Source: CAD feature listing. Evaluate the final solid. Frame: model axes, mm. Coordinates: 2 decimals unless noted, no trailing zeros. Order: outer loops, then holes, each group sorted by start corner. A loop starts at its lowest first (then second) coordinate and runs counter-clockwise, first axis right, second up. Notation, with made-up numbers: (80.5, -35.5) -> (124.5, -35.5) arc R19 ccw to (124.5, -11.5) -> close; hole circle Ø2 at (41, -20.5). An arc over 180 degrees is marked (long way). Put each result on its own line as item: value.
Autodesk Inventor part; units mm, degrees
ref_plane "YZ Plane" through (0, 0, 0) normal (1, 0, 0) x (0, 1, 0)
ref_plane "XZ Plane" through (0, 0, 0) normal (0, 1, 0) x (-1, 0, 0)
ref_plane "XY Plane" through (0, 0, 0) normal (0, 0, 1) x (1, 0, 0)
sketch "Sketch1" plane through (0, 0, 0) normal (0, 0, 1) x (1, 0, 0)
  line L0 (-8.0811, -5.1131) -> (16.9189, -5.1131)
  line L1 (16.9189, -5.1131) -> (16.9189, 19.8869)
  line L2 (16.9189, 19.8869) -> (-8.0811, 19.8869)
  line L3 (-8.0811, 19.8869) -> (-8.0811, -5.1131)
  line L4 (-8.0811, -5.1131) -> (-7.0811, -5.1131)
  line L5 (-7.0811, -5.1131) -> (-7.0811, -4.1131)
  line L6 (-7.0811, -4.1131) -> (-8.0811, -4.1131)
  line L7 (-8.0811, -4.1131) -> (-8.0811, -5.1131)
  line L8 (16.9189, 19.8869) -> (15.9189, 19.8869)
  line L9 (15.9189, 19.8869) -> (15.9189, 18.8869)
  line L10 (15.9189, 18.8869) -> (16.9189, 18.8869)
  line L11 (16.9189, 18.8869) -> (16.9189, 19.8869)
  line L12 (-7.0811, -4.1131) -> (15.9189, -4.1131)
  line L13 (15.9189, -4.1131) -> (15.9189, 18.8869)
  line L14 (15.9189, 18.8869) -> (-7.0811, 18.8869)
  line L15 (-7.0811, 18.8869) -> (-7.0811, -4.1131)
  line L16 (-7.0811, -4.1131) -> (-1.0811, -4.1131)
  line L17 (-1.0811, -4.1131) -> (-1.0811, 17.1845)
  line L18 (-1.0811, 17.1845) -> (-7.0811, 17.1845)
  line L19 (-7.0811, 17.1845) -> (-7.0811, -4.1131)
  line L20 (15.9189, -4.1131) -> (9.9189, -4.1131)
  line L21 (9.9189, -4.1131) -> (9.9189, 17.1845)
  line L22 (9.9189, 17.1845) -> (15.9189, 17.1845)
  line L23 (15.9189, 17.1845) -> (15.9189, -4.1131)
  circle A0 centre (4.4189, 0.3869) radius 5.5
  line L24 (4.4189, 0.3869) -> (15.9189, 0.3869)
  line L25 (4.4189, 0.3869) -> (-8.0811, 0.3869)
  circle A1 centre (-4.0811, 3.3869) radius 3
  circle A2 centre (12.9189, 3.3869) radius 3
  circle A3 centre (4.4189, 0.3869) radius 5
  line L26 (4.4189, -4.6131) -> (4.4189, -3.3131)
  line L27 (4.4189, -3.3131) -> (16.9189, -3.3131)
  line L28 (4.4189, -3.3131) -> (-8.0811, -3.3131)
  line L29 (-4.0811, 6.3869) -> (-4.0811, 8.3869)
  line L30 (-4.0811, 8.3869) -> (16.9189, 8.3869)
  line L31 (-4.0811, 8.3869) -> (-8.0811, 8.3869)
  point P0 (0, 0)
  point P1 (0.3495, -3.3131)
  point P2 (8.4883, -3.3131)
  dimension "d8" = 10
  dimension "d0" = 25
  dimension "d1" = 25
  dimension "d2" = 1
  dimension "d3" = 1
  dimension "d4" = 1
  dimension "d5" = 1
  dimension "d6" = 6
  dimension "d7" = 6
  dimension "d9" = 1.3
  dimension "d10" = 2
extrude "Extrusion1" add sketch "Sketch1" against normal blind 1 contours L3 L25 L15 L28 | L15 L25 L17 L28 | L3 L31 L15 L25 | L27 L13 L30 L1 | L28 L17 A0 | A0 L21 L27 | L15 A1 L25 | L27 L21 L24 L13 | L25 A1 L17 | L17 L30 L21 A0 | L21 A2 L24 | L15 L31 L29 A1 | L13 A2 L21 L30 | L24 A2 L13 | A1 L29 L30 L17
sketch "Sketch3" plane through (0, 0, 0) normal (0, 0, 1) x (1, 0, 0)
  line L0 (-8.0811, 8.3869) -> (-8.0811, -3.3131)
  line L1 (-8.0811, -3.3131) -> (0.3495, -3.3131)
  arc A0 (8.4883, -3.3131) -> (0.3495, -3.3131) centre (4.4189, 0.3869) ccw
  line L2 (8.4883, -3.3131) -> (16.9189, -3.3131)
  line L3 (16.9189, -3.3131) -> (16.9189, 8.3869)
  line L4 (16.9189, 8.3869) -> (-8.0811, 8.3869)
  circle A1 centre (12.9189, 3.3869) radius 3
  circle A2 centre (-4.0811, 3.3869) radius 3
  circle A3 centre (4.4189, 0.3869) radius 1.1
  arc A4 (8.4883, -3.3131) -> (0.3495, -3.3131) centre (4.4189, 0.3869) ccw
  line L5 (16.9189, -3.3131) -> (8.4883, -3.3131)
  line L6 (0.3495, -3.3131) -> (8.4883, -3.3131)
  point P0 (0, 0)
extrude "Extrusion2" add sketch "Sketch3" against normal blind 1 contours A0 L6
sketch "Sketch4" plane through (0, 0, -1) normal (0, 0, -1) x (-1, 0, 0)
  circle A0 centre (-4.4189, 0.3869) radius 1.1
  line L0 (8.0811, -3.3131) -> (8.0811, 8.3869)
  line L1 (8.0811, 8.3869) -> (-16.9189, 8.3869)
  line L2 (-16.9189, 8.3869) -> (-16.9189, -3.3131)
  line L3 (-16.9189, -3.3131) -> (8.0811, -3.3131)
  circle A1 centre (-12.9189, 3.3869) radius 3
  circle A2 centre (4.0811, 3.3869) radius 3
  circle A3 centre (-12.9189, 3.3869) radius 4
  line L4 (-16.9189, 8.3869) -> (-16.9189, -3.3131)
  line L5 (-12.9189, 7.3869) -> (-12.9189, 8.3869)
  line L6 (-12.9189, 7.8869) -> (-16.9189, 7.8869)
  line L7 (-12.9189, 7.8869) -> (8.0811, 7.8869)
  line L8 (8.0811, -3.3131) -> (8.0811, 8.3869)
  point P0 (0, 0)
  point P1 (8.0811, 7.8869)
extrude "Extrusion3" cut sketch "Sketch4" against normal blind 1 contours L7 L5 L1 L0 | L6 L2 L1 L5
fillet "Fillet1" radius 1 4 edges at (16.9189, 7.8869, -0.5) (16.9189, -3.3131, -0.5) (-8.0811, 7.8869, -0.5) (-8.0811, -3.3131, -0.5)
sketch "Sketch5" plane through (0, 0, -1) normal (0, 0, -1) x (-1, 0, 0)
  circle A0 centre (4.0811, 3.3869) radius 3
  circle A1 centre (-12.9189, 3.3869) radius 3
  circle A2 centre (-4.4189, 0.3869) radius 1.1
  arc A3 (7.0811, -3.3131) -> (8.0811, -2.3131) centre (7.0811, -2.3131) ccw
  line L0 (8.0811, -2.3131) -> (8.0811, 6.8869)
  arc A4 (8.0811, 6.8869) -> (7.0811, 7.8869) centre (7.0811, 6.8869) ccw
  line L1 (7.0811, 7.8869) -> (-15.9189, 7.8869)
  arc A5 (-15.9189, 7.8869) -> (-16.9189, 6.8869) centre (-15.9189, 6.8869) ccw
  line L2 (-16.9189, 6.8869) -> (-16.9189, -2.3131)
  arc A6 (-16.9189, -2.3131) -> (-15.9189, -3.3131) centre (-15.9189, -2.3131) ccw
  line L3 (-15.9189, -3.3131) -> (7.0811, -3.3131)
  point P0 (0, 0)
extrude "Extrusion4" add sketch "Sketch5" along normal blind 0.2
sketch "Sketch6" plane through (0, 0, 0) normal (0, 0, 1) x (1, 0, 0)
  arc A0 (-8.0811, -2.3131) -> (-7.0811, -3.3131) centre (-7.0811, -2.3131) ccw
  line L0 (-7.0811, -3.3131) -> (15.9189, -3.3131)
  arc A1 (15.9189, -3.3131) -> (16.9189, -2.3131) centre (15.9189, -2.3131) ccw
  line L1 (16.9189, -2.3131) -> (16.9189, 6.8869)
  arc A2 (16.9189, 6.8869) -> (15.9189, 7.8869) centre (15.9189, 6.8869) ccw
  line L2 (15.9189, 7.8869) -> (-7.0811, 7.8869)
  arc A3 (-7.0811, 7.8869) -> (-8.0811, 6.8869) centre (-7.0811, 6.8869) ccw
  line L3 (-8.0811, 6.8869) -> (-8.0811, -2.3131)
  circle A4 centre (4.4189, 0.3869) radius 1.1
  circle A5 centre (12.9189, 3.3869) radius 3
  circle A6 centre (-4.0811, 3.3869) radius 3
  point P0 (0, 0)
extrude "Extrusion5" add sketch "Sketch6" along normal blind 0.2
properties part number "bok"
1. First-contact query: pin 1 (5.5 mm diameter, centred on x = 12.92, y = 3.39, fed in from +Z). Flat tip, straight axial feed; report the tip coordinate or a pass-through.
Numbers:
pin 1: passes through
2. Cut plane C-C on y = 0.75. Output: boundary loops of the cut face in (x, z), plus the area to 3 significant figures.
Numbers:
outline: (-8.08, -1.2) -> (-5.51, -1.2) -> (-5.51, 0.2) -> (-8.08, 0.2) -> close; (-2.65, -1.2) -> (3.38, -1.2) -> (3.38, 0.2) -> (-2.65, 0.2) -> close; (5.46, -1.2) -> (11.49, -1.2) -> (11.49, 0.2) -> (5.46, 0.2) -> close; (14.35, -1.2) -> (16.92, -1.2) -> (16.92, 0.2) -> (14.35, 0.2) -> close
area: 24.1 mm2
3. Cut plane B-B on x = -6. Output: boundary loops of the cut face in (y, z), plus the area to 3 significant figures.
Numbers:
outline: (-3.31, -1.2) -> (1.08, -1.2) -> (1.08, 0.2) -> (-3.31, 0.2) -> close; (5.69, -1.2) -> (7.89, -1.2) -> (7.89, 0.2) -> (5.69, 0.2) -> close
area: 9.22 mm2
4. Ray query, line 1 along X through (y, z) = (2, -0.1); line 2 along Y through (x, z) = (-4.25, -0.55); line 3 along X through (y, z) = (2.25, -0.95). Return the intervals inside material, ascending.
Numbers:
line 1: x = -8.08 to -6.74, -1.42 to 10.26, 15.58 to 16.92
line 2: y = -3.31 to 0.39, 6.38 to 7.89
line 3: x = -8.08 to -6.86, -1.3 to 10.14, 15.7 to 16.92
5. Pull-direction query (Y, two-part tool) for faces 1 (the flat face through (16.919, 2, -1)), 2 (the flat face through (4, -3.313, -1)), 3 (the cylindrical face through (-7.796, 7.586, -0.51)), 4 (the cylindrical face through (13.12, 6.38, -0.49)); classes: pulls with the +Y half, pulls with the -Y half, needs draft (parallel to the pull), parting line crosses it, or undercut.
Numbers:
face 1: needs draft
face 2: pulls with the -Y half
face 3: pulls with the +Y half
face 4: undercut
6. Cut plane D-D on z = -0.7. Output: boundary loops of the cut face in (x, y).
Numbers:
outline: (-8.08, -2.31) arc R1 ccw to (-7.08, -3.31) -> (15.92, -3.31) arc R1 ccw to (16.92, -2.31) -> (16.92, 6.89) arc R1 ccw to (15.92, 7.89) -> (-7.08, 7.89) arc R1 ccw to (-8.08, 6.89) -> close; hole circle Ø6 at (-4.08, 3.39); hole circle Ø2.2 at (4.42, 0.39); hole circle Ø6 at (12.92, 3.39)
7. Cut plane A-A on y = 5.5. Output: boundary loops of the cut face in (x, z), plus the area to 3 significant figures.
Numbers:
outline: (-8.08, -1.2) -> (-6.21, -1.2) -> (-6.21, 0.2) -> (-8.08, 0.2) -> close; (-1.95, -1.2) -> (10.79, -1.2) -> (10.79, 0.2) -> (-1.95, 0.2) -> close; (15.05, -1.2) -> (16.92, -1.2) -> (16.92, 0.2) -> (15.05, 0.2) -> close
area: 23.1 mm2
